Model file for the job. Use its own axes, mm. A direction names the side the tool comes from. Coordinates: 2 decimals unless noted, no trailing zeros. Order: outer loops, then holes, each group sorted by start corner. A loop starts at its lowest first (then second) coordinate and runs counter-clockwise, first axis right, second up. Notation, with made-up numbers: (21.25, 18) -> (72.25, 18) arc R22 cw to (72.25, 45) -> close; hole circle Ø4 at (37.25, -35.5). An arc over 180 degrees is marked (long way). Use CSV: the item, a comma, the result in double quotes. Start each with the question number.
(1) Pin check, flat tips, straight feed: pin 1 Ø3 at (x, y) = (-10, 28) entering from -Z; pin 2 Ø4.5 at (x, z) = (25, -25) entering from +Y; pin 3 Ø22 at (y, z) = (44.5, -3.5) entering from -X; pin 4 Ø13 at (y, z) = (46.5, -1) entering from +X. Stop position of each tip, or through.
(2) Cut at A-A on z = 25. Write the cut outline in (x, y).
(3) Tool access for faces 1 (the flat face through (-10.05, 35, 0)), 2 (the flat face through (0, 0, 0)), 3 (the cylindrical face through (-14.48, 35.42, 14.45)): list every direction of +Z, -Z, +X, -X, +Y, -Y with a clear straight run to the whole face (end or side of a thin tool).
(4) Cut at C-C on y = 48. Write the cut outline in (x, z).
(5) Cut at B-B on x = 25. Write the cut outline in (y, z), plus the area to 3 significant figures.
(6) Probe L1, parallel to X at y = 2, z = 25; L2, parallel to X at y = 6, z = 3. List the from-to ranges inside material, lowest first.
(7) Pull direction X, two halves, no side cores. Call faces 4 (the flat face through (0, 1, -31)), 5 (the cylindrical face through (-30.43, 1.52, 30.4)), 6 (the flat face through (10.05, 35, 0)): pulls with the +X half, pulls with the -X half, needs draft (parallel to the pull), parting line crosses it, or undercut.
(8) Cut at D-D on z = 2. Write the cut outline in (x, y).
Autodesk Inventor part; units mm, degrees
ref_plane "YZ Plane" through (0, 0, 0) normal (1, 0, 0) x (0, 1, 0)
ref_plane "XZ Plane" through (0, 0, 0) normal (0, 1, 0) x (-1, 0, 0)
ref_plane "XY Plane" through (0, 0, 0) normal (0, 0, 1) x (1, 0, 0)
sketch "스케치2" plane through (0, 0, 0) normal (0, 1, 0) x (-1, 0, 0)
  line L0 (25, 25) -> (-25, 25)
  line L1 (-25, 25) -> (-25, -25)
  line L2 (-25, -25) -> (25, -25)
  line L3 (25, -25) -> (25, 25)
  line L4 (25, 25) -> (-25, -25) construction
  line L5 (-25, 25) -> (25, -25) construction
  circle A0 centre (25, -25) radius 2.6
  circle A1 centre (-25, -25) radius 2.6
  circle A2 centre (25, 25) radius 2.6
  circle A3 centre (-25, 25) radius 2.6
  line L6 (31, -31) -> (-31, -31)
  line L7 (-31, -31) -> (-31, 31)
  line L8 (-31, 31) -> (31, 31)
  line L9 (31, 31) -> (31, -31)
  line L10 (10.05, 10.05) -> (-10.05, 10.05)
  line L11 (-10.05, 10.05) -> (-10.05, -10.05)
  line L12 (-10.05, -10.05) -> (10.05, -10.05)
  line L13 (10.05, -10.05) -> (10.05, 10.05)
  line L14 (10.05, 10.05) -> (-10.05, -10.05) construction
  line L15 (-10.05, 10.05) -> (10.05, -10.05) construction
  line L16 (-15.05, -15.05) -> (-15.05, 15.05)
  line L17 (-15.05, 15.05) -> (15.05, 15.05)
  line L18 (15.05, 15.05) -> (15.05, -15.05)
  line L19 (15.05, -15.05) -> (-15.05, -15.05)
  point P0 (0, 0)
  dimension "d16" = 50
  dimension "d17" = 50
  dimension "d18" = 5.2
  dimension "d21" = 50
  dimension "d24" = 50
  dimension "d27" = 6
  dimension "d28" = 20.1
  dimension "d29" = 20.1
  dimension "d30" = 5
extrude "돌출2" add sketch "스케치2" along normal blind 5 contours L0 A2 L3 A0 L2 A1 L1 A3 | L6 L7 L8 L9 | L13 L12 L11 L10 | L16 L17 L18 L19
sketch "스케치3" plane through (0, 5, 0) normal (0, 1, 0) x (1, 0, 0)
  line L0 (-10.05, 10.05) -> (10.05, 10.05)
  line L1 (10.05, 10.05) -> (10.05, -10.05)
  line L2 (10.05, -10.05) -> (-10.05, -10.05)
  line L3 (-10.05, -10.05) -> (-10.05, 10.05)
  line L4 (-10.05, 10.05) -> (10.05, -10.05) construction
  line L5 (10.05, 10.05) -> (-10.05, -10.05) construction
  line L6 (15.05, 15.05) -> (-15.05, 15.05)
  line L7 (-15.05, 15.05) -> (-15.05, -15.05)
  line L8 (-15.05, -15.05) -> (15.05, -15.05)
  line L9 (15.05, -15.05) -> (15.05, 15.05)
  point P0 (0, 0)
  dimension "d33" = 20.1
  dimension "d34" = 20.1
  dimension "d35" = 5
extrude "돌출3" add sketch "스케치3" along normal blind 60
fillet "모깎기1" radius 2 12 edges at (-31, 5, 0) (0, 5, -31) (0, 5, 31) (31, 5, 0) (-31, 2.5, -31) (-31, 2.5, 31) (31, 2.5, 31) (31, 2.5, -31) (-15.05, 35, 15.05) (15.05, 35, 15.05) (15.05, 35, -15.05) (-15.05, 35, -15.05)
properties part number "Profile_Holder"
Outcome:
1,pin 1,"z = -15.05"
1,pin 2,"through"
1,pin 3,"x = -15.05"
1,pin 4,"x = 15.05"
2,outline,"(-31, 0) -> (-27.6, 0) -> (-27.6, 5) -> (-29, 5) arc R2 ccw to (-31, 3) -> close; (-22.4, 0) -> (22.4, 0) -> (22.4, 5) -> (-22.4, 5) -> close; (27.6, 0) -> (31, 0) -> (31, 3) arc R2 ccw to (29, 5) -> (27.6, 5) -> close"
3,face 1,"+Y"
3,face 2,"+Z, -Z, +X, -X, -Y"
3,face 3,"+Z, -X, +Y"
4,outline,"(-15.05, -13.05) arc R2 ccw to (-13.05, -15.05) -> (13.05, -15.05) arc R2 ccw to (15.05, -13.05) -> (15.05, 13.05) arc R2 ccw to (13.05, 15.05) -> (-13.05, 15.05) arc R2 ccw to (-15.05, 13.05) -> close; hole (-10.05, -10.05) -> (10.05, -10.05) -> (10.05, 10.05) -> (-10.05, 10.05) -> close"
5,outline,"(0, -31) -> (3, -31) arc R2 ccw to (5, -29) -> (5, -27.6) -> (0, -27.6) -> close; (0, -22.4) -> (5, -22.4) -> (5, 22.4) -> (0, 22.4) -> close; (0, 27.6) -> (5, 27.6) -> (5, 29) arc R2 ccw to (3, 31) -> (0, 31) -> close"
5,area,"256 mm2"
6,L1,"-31 to -27.6, -22.4 to 22.4, 27.6 to 31"
6,L2,"-15.05 to -10.05, 10.05 to 15.05"
7,face 4,"needs draft"
7,face 5,"pulls with the -X half"
7,face 6,"undercut"
8,outline,"(-31, 0) -> (31, 0) -> (31, 3) arc R2 ccw to (29, 5) -> (15.05, 5) -> (15.05, 65) -> (10.05, 65) -> (10.05, 5) -> (-10.05, 5) -> (-10.05, 65) -> (-15.05, 65) -> (-15.05, 5) -> (-29, 5) arc R2 ccw to (-31, 3) -> close"
